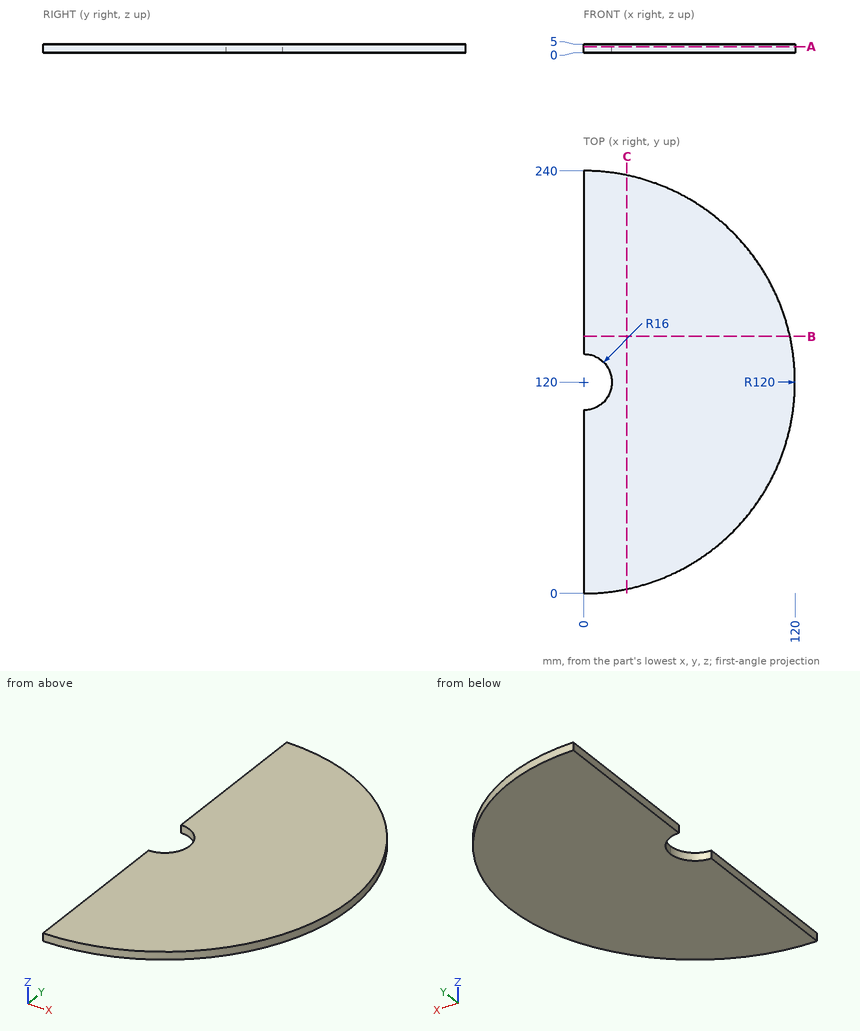
Verification items for this drawing (mm, ordinates from the low corner). Coordinates: 2 decimals unless noted, no trailing zeros. Write each loop counter-clockwise with the first axis right and the second up, starting at its lowest first coordinate (ties: lowest second). Pieces come first, ordered by that corner, then holes. Notation, with made-up numbers: M 34,86.25 L 80,86.25 A16 cw 80,90.25 Z; hole C 7.5,51.25 d1. An arc over 180 degrees is marked long. Answer as a JSON object with one key per item and string values. Group by question number.
(1) Material ranges on line 1 (Y direction, x = 13.5, z = 0.65); line 2 (X direction, y = 201.5, z = 1.1); line 3 (X direction, y = 83, z = 2.4), recorded low to high.
(2) Gauge pin test, flat ends, axial feed: pin 1 (3 mm diameter, centred on x = 98, z = 0.5, fed in from -Y); pin 2 (2 mm diameter, centred on x = 84.5, z = 4, fed in from -Y). Record the tip position at first contact, or that the pin passes through.
(3) Cross-section at A-A, the plane z = 3.45. Record the cut outline in (x, y).
(4) Cross-section at B-B, the plane y = 146. Record the cut outline in (x, z), and give its area (3 significant figures).
(5) Cross-section at C-C, the plane x = 24.5. Record the cut outline in (y, z).
Reply:
{
 "1": {"line 1": "0.76 to 111.41, 128.59 to 239.24", "line 2": "0 to 88.08", "line 3": "0 to 114.15"},
 "2": {"pin 1": "y = 48.67", "pin 2": "y = 33.82"},
 "3": {"outline": "M 0,0 A120 ccw 0,240 L 0,136 A16 cw 0,104 Z"},
 "4": {"outline": "M 0,0 L 117.15,0 L 117.15,5 L 0,5 Z", "area": "586 mm²"},
 "5": {"outline": "M 2.53,0 L 237.47,0 L 237.47,5 L 2.53,5 Z"}
}
